Source: three-view drawing plus pictorial views. Frame: mm from the lowest corner of the part. A direction names the side the tool comes from. Coordinates: 2 decimals unless noted, no trailing zeros. Order: outer loops, then holes, each group sorted by start corner. A loop starts at its lowest first (then second) coordinate and runs counter-clockwise, first axis right, second up. Notation, with made-up numbers: (24, 74) -> (36, 74) arc R34 ccw to (36, 109) -> close; hole circle Ø2 at (-2.5, -21). An arc over 180 degrees is marked (long way). Use one line per item in the form item = value. Start each with the question number.
1) Section query B-B on z = 5. Output: boundary loops of the cut face in (x, y), then the cut area to 3 significant figures.
2) Section query D-D on z = 18.75. Output: boundary loops of the cut face in (x, y).
3) Pin query (flat end, axial travel): pin 1 (2 mm diameter, centred on x = 15, z = 13, fed in from +Y); pin 2 (3 mm diameter, centred on y = 38.5, z = 13, fed in from +X); pin 3 (4 mm diameter, centred on y = 22.5, z = 15, fed in from -X); pin 4 (5.5 mm diameter, centred on x = 16.5, z = 14, fed in from -Y). Return the tip coordinate at first contact, or that it passes through.
4) Ray query, line 1 along X through (y, z) = (22.5, 12); line 2 along Y through (x, z) = (2.75, 5); line 3 along Z through (x, y) = (4.5, 22). Return the intervals inside material, ascending.
5) Draft query along X for the marked faces 1, 2 and 3. Return one class per face: pulls with the +X half, pulls with the -X half, needs draft (parallel to the pull), parting line crosses it, or undercut.
6) Section query C-C on x = 16.25. Output: boundary loops of the cut face in (y, z).
7) Access query for the marked faces 4, 5, 6, 7 and 8. Directions: +Z, -Z, +X, -X, +Y, -Y. A direction counts if a zero-diameter tool reaches every point of the face in a straight line with its end or side. Return the directions, or none.
8) Section query A-A on y = 22.5. Output: boundary loops of the cut face in (x, z).
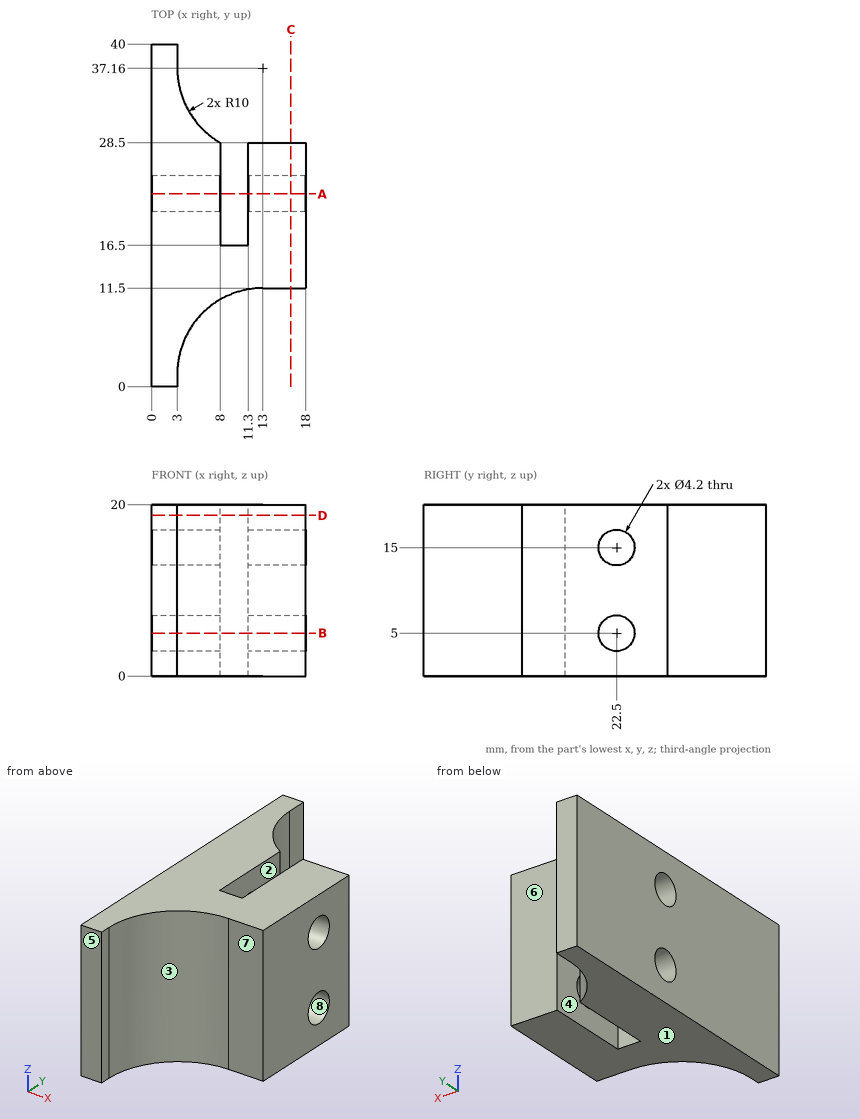
Answers below:
q1.outline = (0, 0) -> (3, 0) -> (3, 1.5) arc R10 cw to (13, 11.5) -> (18, 11.5) -> (18, 20.4) -> (11.3, 20.4) -> (11.3, 16.5) -> (8, 16.5) -> (8, 20.4) -> (0, 20.4) -> close; (0, 24.6) -> (8, 24.6) -> (8, 28.5) arc R10 cw to (3, 37.16) -> (3, 40) -> (0, 40) -> close; (11.3, 24.6) -> (18, 24.6) -> (18, 28.5) -> (11.3, 28.5) -> close
q1.area = 308 mm^2
q2.outline = (0, 0) -> (3, 0) -> (3, 1.5) arc R10 cw to (13, 11.5) -> (18, 11.5) -> (18, 28.5) -> (11.3, 28.5) -> (11.3, 16.5) -> (8, 16.5) -> (8, 28.5) arc R10 cw to (3, 37.16) -> (3, 40) -> (0, 40) -> close
q3.pin_1 = 28.5
q3.pin_2 = 3
q3.pin_3 = through
q3.pin_4 = 11.5
q4.line_1 = 0 to 8, 11.3 to 18
q4.line_2 = 0 to 20.4, 24.6 to 40
q4.line_3 = 0 to 2.96, 7.04 to 12.96, 17.04 to 20
q5.face_1 = needs draft
q5.face_2 = undercut
q5.face_3 = pulls with the +X half
q6.outline = (11.5, 0) -> (28.5, 0) -> (28.5, 20) -> (11.5, 20) -> close; hole circle Ø4.2 at (22.5, 5); hole circle Ø4.2 at (22.5, 15)
q7.face_4 = +Z, -Z, +Y
q7.face_5 = +Z, -Z, +X, -X, -Y
q7.face_6 = +Z, -Z, +X, +Y
q7.face_7 = +Z, -Z, +X, -Y
q7.face_8 = +X, -X
q8.outline = (0, 0) -> (8, 0) -> (8, 2.9) -> (0, 2.9) -> close; (0, 7.1) -> (8, 7.1) -> (8, 12.9) -> (0, 12.9) -> close; (0, 17.1) -> (8, 17.1) -> (8, 20) -> (0, 20) -> close; (11.3, 0) -> (18, 0) -> (18, 2.9) -> (11.3, 2.9) -> close; (11.3, 7.1) -> (18, 7.1) -> (18, 12.9) -> (11.3, 12.9) -> close; (11.3, 17.1) -> (18, 17.1) -> (18, 20) -> (11.3, 20) -> close
